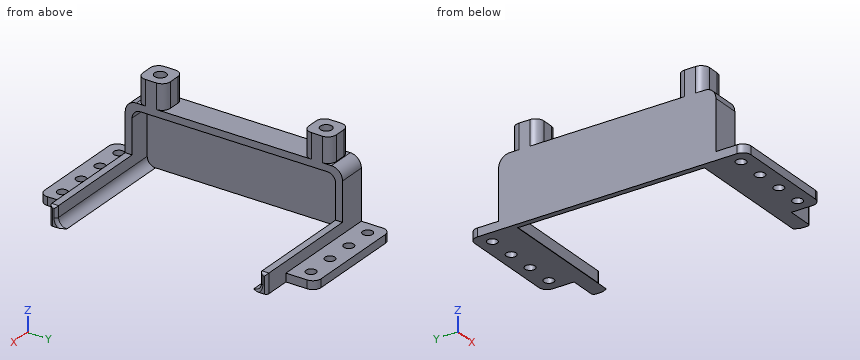
from build123d import *

# Parameters (mm, degrees)
BOX_W             = 141
BOX_H             = 73.6
BOX_DEPTH         = 22.5
FILLET_R          = 3
CYLINDER001_R     = 2.1
CYLINDER001_DEPTH = 10
BOX003_W          = 10
BOX003_H          = 10
BOX003_DEPTH      = 9
FILLET003_R       = 3
CYLINDER_R        = 1.8
CYLINDER_DEPTH    = 10
ARRAY_X_COUNT     = 4
ARRAY_X_PITCH     = 10
BOX002_W          = 40
BOX002_H          = 100
BOX002_DEPTH      = 3
FILLET001_R       = 3
BOX005_W          = 50
BOX005_H          = 78.6
BOX005_DEPTH      = 7
FILLET005_R       = 1
BOX001_W          = 10
BOX001_H          = 78.6
BOX001_DEPTH      = 25
FILLET002_R       = 4


with BuildPart() as battery_fillet:
    # Box → Box (new body)
    with BuildSketch(Plane(origin=(2, 0, 0), x_dir=(1, 0, 0), z_dir=(0, 0, 1))):
        with Locations((70.5, 36.8)):
            Rectangle(BOX_W, BOX_H)
    extrude(amount=BOX_DEPTH)

    # Fillet
    fillet_edges = [battery_fillet.edges().sort_by_distance(p)[0] for p in [
        (72.5, 0, 0),
        (72.5, 0, 22.5),
        (72.5, 73.6, 0),
        (72.5, 73.6, 22.5),
    ]]
    fillet(fillet_edges, radius=FILLET_R)


with BuildPart() as battery_fillet_1:
    # Fillet placement: moved
    add(battery_fillet.part.moved(Location((0, -36.8, 0))))


with BuildPart() as insert_hole:
    # Cylinder001 → Cylinder001 (new body)
    with BuildSketch(Plane(origin=(5, 0, 0), x_dir=(1, 0, 0), z_dir=(0, 0, 1))):
        Circle(CYLINDER001_R)
    extrude(amount=CYLINDER001_DEPTH)


with BuildPart() as top_insert_box_cut:
    # Box003 → Box003 (new body)
    with BuildSketch(Plane(origin=(0, -5, 0), x_dir=(1, 0, 0), z_dir=(0, 0, 1))):
        with Locations((5, 5)):
            Rectangle(BOX003_W, BOX003_H)
    extrude(amount=BOX003_DEPTH)

    # Fillet003
    fillet003_edges = [top_insert_box_cut.edges().sort_by_distance(p)[0] for p in [
        (0, -5, 4.5),
        (0, 5, 4.5),
        (10, -5, 4.5),
        (10, 5, 4.5),
    ]]
    fillet(fillet003_edges, radius=FILLET003_R)

    # Cut: cut insert hole
    add(insert_hole.part, mode=Mode.SUBTRACT)


with BuildPart() as top_insert_box_cut_1:
    # Cut placement: moved
    add(top_insert_box_cut.part.moved(Location((0, 30, 25))))


with BuildPart() as part_mirroring001:
    # Part__Mirroring001: instance of top insert box cut
    add(top_insert_box_cut_1.part.mirror(Plane(origin=(0, 0, 0), x_dir=(1, 0, 0), z_dir=(0, 1, 0))))


with BuildPart() as bolt_hole:
    # Cylinder → Cylinder (new body)
    with BuildSketch(Plane(origin=(5, 45, 0), x_dir=(1, 0, 0), z_dir=(0, 0, 1))):
        Circle(CYLINDER_R)
    extrude(amount=CYLINDER_DEPTH)


with BuildPart() as bolt_hole_array:
    # Part__Mirroring: instance of bolt hole
    add(bolt_hole.part.mirror(Plane(origin=(0, 0, 0), x_dir=(1, 0, 0), z_dir=(0, 1, 0))))

    # Fusion: union bolt hole
    add(bolt_hole.part)

    # Array X: bolt hole array ×4


with BuildPart() as bolt_hole_array_1:
    add(bolt_hole_array.part)
    with Locations(*[(i * ARRAY_X_PITCH, 0, 0) for i in range(1, ARRAY_X_COUNT)]):
        add(bolt_hole_array.part)


with BuildPart() as back_wall_bottom_cut:
    # Box002 → Box002 (new body)
    with BuildSketch(Plane(origin=(0, -50, 0), x_dir=(1, 0, 0), z_dir=(0, 0, 1))):
        with Locations((20, 50)):
            Rectangle(BOX002_W, BOX002_H)
    extrude(amount=BOX002_DEPTH)

    # Fillet001
    fillet001_edges = [back_wall_bottom_cut.edges().sort_by_distance(p)[0] for p in [
        (0, -50, 1.5),
        (0, 50, 1.5),
        (40, -50, 1.5),
        (40, 50, 1.5),
    ]]
    fillet(fillet001_edges, radius=FILLET001_R)

    # Cut001: cut bolt hole array
    add(bolt_hole_array_1.part, mode=Mode.SUBTRACT)


with BuildPart() as big_bottom_cube_fillet:
    # Box005 → Box005 (new body)
    with BuildSketch(Plane(origin=(0, -39.3, 0), x_dir=(1, 0, 0), z_dir=(0, 0, 1))):
        with Locations((25, 39.3)):
            Rectangle(BOX005_W, BOX005_H)
    extrude(amount=BOX005_DEPTH)

    # Cut004: cut battery fillet
    add(battery_fillet_1.part, mode=Mode.SUBTRACT)

    # Fillet005
    fillet005_edges = [big_bottom_cube_fillet.edges().sort_by_distance(p)[0] for p in [
        (50, -39.3, 3.5),
        (50, 38.05, 7),
        (50, -38.05, 7),
        (50, 39.3, 3.5),
        (50, -36.8, 5),
        (50, -35.92132, 0.87868),
        (50, 35.92132, 0.87868),
        (50, 36.8, 5),
    ]]
    fillet(fillet005_edges, radius=FILLET005_R)


with BuildPart() as battery_back_wall_cut:
    # Box001 → Box001 (new body)
    with BuildSketch(Plane(origin=(0, -39.3, 0), x_dir=(1, 0, 0), z_dir=(0, 0, 1))):
        with Locations((5, 39.3)):
            Rectangle(BOX001_W, BOX001_H)
    extrude(amount=BOX001_DEPTH)

    # Fillet002
    fillet002_edges = [battery_back_wall_cut.edges().sort_by_distance(p)[0] for p in [
        (5, -39.3, 25),
        (5, 39.3, 25),
    ]]
    fillet(fillet002_edges, radius=FILLET002_R)

    # Fusion001: union Part__Mirroring001, top insert box cut, back wall bottom cut, big bottom cube fillet
    add(part_mirroring001.part)
    add(top_insert_box_cut_1.part)
    add(back_wall_bottom_cut.part)
    add(big_bottom_cube_fillet.part)

    # Cut002: cut battery fillet
    add(battery_fillet_1.part, mode=Mode.SUBTRACT)


solid = battery_back_wall_cut.part
Design review of the part built by this model. Coordinates are the model's own, in mm. Round coordinates to 2 decimals unless told otherwise and drop trailing zeros. Write each loop counter-clockwise with the first axis right and the second up, starting at its lowest first coordinate (ties: lowest second). Pieces come first, ordered by that corner, then holes. Notation, with made-up numbers: (78, 74.25) -> (130, 74.25) arc R20 ccw to (130, 87.25) -> close; hole circle Ø5 at (-10, 80). An arc over 180 degrees is marked (long way). One line per item, written item: value. Start each with the question number.
Q1. To check wall thickness, follow probe 1 along X at (y, z) = (-45, 1); probe 2 along Y at (x, z) = (3.5, 17); probe 3 along Y at (x, z) = (25, 2.3). State the ranges of each line that lie inside material, in increasing order.
Q2. Add section B-B (x = 47). Give the boundary of the cut face in (y, z), then the cut area to 3 significant figures.
Q3. Add section D-D (x = 15). Give the boundary of the cut face in (y, z).
Q4. Add section A-A (z = 31). Give the boundary of the cut face in (x, y).
Q5. Add section C-C (y = 45). Give the boundary of the cut face in (x, z).
Q6. Insertion check: P1, Ø5, axis at x = 44, z = 6, coming from the +Y side; P2, Ø3, axis at x = 35, y = -45, coming from the +Z side; P3, Ø4.5, axis at x = 4.5, z = 30.5, coming from the +Y side; P4, Ø8, axis at y = -36.5, z = 27.5, coming from the +X side. Each pin has a flat end and moves straight along its axis. Give the tip position at first contact, or say it passes through.
Response:
1. probe 1: x = 0 to 3.2, 6.8 to 13.2, 16.8 to 23.2, 26.8 to 33.2, 36.8 to 40
1. probe 2: y = -39.3 to -36.8, 36.8 to 39.3
1. probe 3: y = -50 to -46.8, -43.2 to -36.72, 36.72 to 43.2, 46.8 to 50
2. outline: (-39.3, 0) -> (-33.8, 0) arc R3 cw to (-36.8, 3) -> (-36.8, 7) -> (-39.3, 7) -> close; (33.8, 0) -> (39.3, 0) -> (39.3, 7) -> (36.8, 7) -> (36.8, 3) arc R3 cw to start
2. area: 38.9 mm^2
3. outline: (-50, 0) -> (-46.8, 0) -> (-46.8, 3) -> (-50, 3) -> close; (-43.2, 0) -> (-33.8, 0) arc R3 cw to (-36.8, 3) -> (-36.8, 7) -> (-39.3, 7) -> (-39.3, 3) -> (-43.2, 3) -> close; (33.8, 0) -> (43.2, 0) -> (43.2, 3) -> (39.3, 3) -> (39.3, 7) -> (36.8, 7) -> (36.8, 3) arc R3 cw to start; (46.8, 0) -> (50, 0) -> (50, 3) -> (46.8, 3) -> close
4. outline: (0, -32) arc R3 ccw to (3, -35) -> (7, -35) arc R3 ccw to (10, -32) -> (10, -28) arc R3 ccw to (7, -25) -> (3, -25) arc R3 ccw to (0, -28) -> close; (0, 28) arc R3 ccw to (3, 25) -> (7, 25) arc R3 ccw to (10, 28) -> (10, 32) arc R3 ccw to (7, 35) -> (3, 35) arc R3 ccw to (0, 32) -> close; hole circle Ø4.2 at (5, -30); hole circle Ø4.2 at (5, 30)
5. outline: (0, 0) -> (3.2, 0) -> (3.2, 3) -> (0, 3) -> close; (6.8, 0) -> (13.2, 0) -> (13.2, 3) -> (6.8, 3) -> close; (16.8, 0) -> (23.2, 0) -> (23.2, 3) -> (16.8, 3) -> close; (26.8, 0) -> (33.2, 0) -> (33.2, 3) -> (26.8, 3) -> close; (36.8, 0) -> (40, 0) -> (40, 3) -> (36.8, 3) -> close
6. P1: stops at y = 39.3
6. P2: passes through
6. P3: stops at y = 35
6. P4: stops at x = 10
